Here's how the part is built. I have some questions about the finished solid (model axes, mm). A direction names the side the tool comes from. Coordinates: 2 decimals unless noted, no trailing zeros. Write each loop counter-clockwise with the first axis right and the second up, starting at its lowest first coordinate (ties: lowest second). Pieces come first, ordered by that corner, then holes. Notation, with made-up numbers: M -8.75,47 L 22.25,47 A29 ccw 22.25,84 Z; hole C -35.5,86.25 d11. An arc over 180 degrees is marked long. Use a Markdown table: item, result.
```python
from build123d import *

# Parameters (mm, degrees)
SKETCH_W            = 194
SKETCH_H            = 191
PAD_DEPTH           = 12
SKETCH002_W         = 180.5
SKETCH002_H         = 184
POCKET_DEPTH        = 11
SKETCH004_W         = 120
SKETCH004_H         = 5
SKETCH004_W_2       = 5
SKETCH004_H_2       = 120
SKETCH004_H_3       = 80
PAD001_DEPTH        = 20
SKETCH005_W         = 72
SKETCH005_H         = 54
PAD002_DEPTH        = 10
SKETCH006_W         = 70
SKETCH006_H         = 50
POCKET001_DEPTH     = 10
SKETCH007_W         = 27
SKETCH007_H         = 3
POCKET002_DEPTH     = 5
SKETCH008_W         = 2.5
SKETCH008_H         = 27
POCKET003_DEPTH     = 5
SKETCH009_W         = 45
SKETCH009_H         = 3
POCKET004_DEPTH     = 5
LINEARPATTERN_COUNT = 4
LINEARPATTERN_PITCH = 5


with BuildPart() as part:
    # Sketch → Pad (new body)
    with BuildSketch(Plane.XY):
        with Locations((97, 95.5)):
            Rectangle(SKETCH_W, SKETCH_H)
    extrude(amount=-PAD_DEPTH)

    # Sketch002 → Pocket (cut)
    with BuildSketch(Plane.XY):
        with Locations((93.75, 95.5)):
            Rectangle(SKETCH002_W, SKETCH002_H)
    extrude(amount=-POCKET_DEPTH, mode=Mode.SUBTRACT)

    # Sketch004 (on Face11 of Pocket) → Pad001 (join)
    with BuildSketch(Plane.XY.offset(-11)):
        with Locations((100, 185)):
            Rectangle(SKETCH004_W, SKETCH004_H)
        with Locations((100, 6)):
            Rectangle(SKETCH004_W, SKETCH004_H)
        with Locations((181.5, 100)):
            Rectangle(SKETCH004_W_2, SKETCH004_H_2)
        with Locations((6, 115.5)):
            Rectangle(SKETCH004_W_2, SKETCH004_H_3)
    extrude(amount=PAD001_DEPTH)

    # Sketch005 (on Face20 of Pad001) → Pad002 (join)
    with BuildSketch(Plane.XY.offset(-11)):
        with Locations((44.5, 42)):
            Rectangle(SKETCH005_W, SKETCH005_H)
    extrude(amount=PAD002_DEPTH)

    # Sketch006 (on Face40 of Pad002) → Pocket001 (cut)
    with BuildSketch(Plane.XY.offset(-1)):
        with Locations((42, 42)):
            Rectangle(SKETCH006_W, SKETCH006_H)
    extrude(amount=-POCKET001_DEPTH, mode=Mode.SUBTRACT)

    # Sketch007 (on Face2 of Pocket001) → Pocket002 (cut)
    with BuildSketch(Plane(origin=(0, 0, 0), x_dir=(0, -1, 0), z_dir=(-1, 0, 0))):
        with Locations((-42.5, -1.5)):
            Rectangle(SKETCH007_W, SKETCH007_H)
    extrude(amount=-POCKET002_DEPTH, mode=Mode.SUBTRACT)

    # Sketch008 (on Face7 of Pocket002) → Pocket003 (cut)
    with BuildSketch(Plane.XY.offset(-3)):
        with Locations((2.25, 42.5)):
            Rectangle(SKETCH008_W, SKETCH008_H)
    extrude(amount=-POCKET003_DEPTH, mode=Mode.SUBTRACT)

    # Sketch009 (on Face22 of Pocket003) → Pocket004 (cut)
    with BuildSketch(Plane.XY.offset(-11)):
        with Locations((101.5, 155.868176)):
            Rectangle(SKETCH009_W, SKETCH009_H)
    pocket004 = extrude(amount=-POCKET004_DEPTH, mode=Mode.SUBTRACT)

    # LinearPattern: Pocket004 ×4
    with Locations(*[(0, -i * LINEARPATTERN_PITCH, 0) for i in range(1, LINEARPATTERN_COUNT)]):
        add(pocket004, mode=Mode.SUBTRACT)


solid = part.part
```
1. We'd pull the mould along X, two halves only. Please class faces 5 (the face through (99, 185, 9)), 6 (the face through (21, 187.5, -5)), 7 (the face through (184, 99, 4)): +X half, -X half, draft (parallel to the pull), parting line (faces both ways), or undercut.
Answers follow:
| item | result |
|---|---|
| face 5 | draft |
| face 6 | undercut |
| face 7 | +X half |
2. Suppose I cut it at C-C on y = 128. Write out the boundary of the cut face in (x, z), and give its area (4 significant figures).
Answers follow:
| item | result |
|---|---|
| outline | M 0,-12 L 194,-12 L 194,0 L 184,0 L 184,9 L 179,9 L 179,-11 L 8.5,-11 L 8.5,9 L 3.5,9 L 3.5,0 L 0,0 Z |
| area | 542.5 mm2 |
3. Which directions (+Z, -Z, +X, -X, +Y, -Y) give clear straight access to the entire face, cutting with the end or side of a thin tool? Please do faces 1 (the face through (99, 187.5, 4)), 2 (the face through (99, 3.5, 4)), 3 (the face through (3.5, 115, 4)), 4 (the face through (184, 21, -5)).
Answers follow:
| item | result |
|---|---|
| face 1 | +Z, +X, -X, +Y |
| face 2 | +Z, +X, -X, -Y |
| face 3 | +Z, -X, +Y, -Y |
| face 4 | +Z |
4. Will this pin go through, and if not, where does the flat tip stop? pin 1 Ø5.5 at (y, z) = (184.5, 2) entering from -X.
Answers follow:
| item | result |
|---|---|
| pin 1 | stops at x = 0 |
5. Suppose I cut it at B-B on z = 5. Write out the boundary of the cut face in (x, y).
Answers follow:
| item | result |
|---|---|
| outline | M 3.5,75.5 L 8.5,75.5 L 8.5,155.5 L 3.5,155.5 Z; M 40,3.5 L 160,3.5 L 160,8.5 L 40,8.5 Z; M 40,182.5 L 160,182.5 L 160,187.5 L 40,187.5 Z; M 179,40 L 184,40 L 184,160 L 179,160 Z |
6. Suppose I cut it at D-D on x = 169. Write out the boundary of the cut face in (y, z), and give its area (3 significant figures).
Answers follow:
| item | result |
|---|---|
| outline | M 0,-12 L 191,-12 L 191,0 L 187.5,0 L 187.5,-11 L 3.5,-11 L 3.5,0 L 0,0 Z |
| area | 268 mm2 |
7. I need wall thicknesses on probe 1 along Y at (x, z) = (61.5, -4.25); probe 2 along X at (y, z) = (67, -0.25); probe 3 along Y at (x, z) = (94.5, -2.5). Which ranges of each line are inside material? Lowest first, please.
Answers follow:
| item | result |
|---|---|
| probe 1 | y = 0 to 8.5, 15 to 17, 67 to 69, 182.5 to 191 |
| probe 2 | x = 0 to 3.5, 179 to 194 |
| probe 3 | y = 0 to 8.5, 182.5 to 191 |
8. Suppose I cut it at A-A on x = 88. Write out the boundary of the cut face in (y, z), and give its area (3 significant figures).
Answers follow:
| item | result |
|---|---|
| outline | M 0,-12 L 139.37,-12 L 139.37,-11 L 8.5,-11 L 8.5,9 L 3.5,9 L 3.5,0 L 0,0 Z; M 142.37,-12 L 144.37,-12 L 144.37,-11 L 142.37,-11 Z; M 147.37,-12 L 149.37,-12 L 149.37,-11 L 147.37,-11 Z; M 152.37,-12 L 154.37,-12 L 154.37,-11 L 152.37,-11 Z; M 157.37,-12 L 191,-12 L 191,0 L 187.5,0 L 187.5,9 L 182.5,9 L 182.5,-11 L 157.37,-11 Z |
| area | 456 mm2 |
